```python
from build123d import *

# Parameters (mm, degrees)
F1_DEPTH = 405
F2_R     = 2.5
F2_R_2   = 4
F3_DEPTH = 2.001
F4_R     = 4
F5_DEPTH = 2.001


with BuildPart() as f1:
    # F0 (on Top) → F1 (new body)
    with BuildSketch(Plane.XY):
        with BuildLine():
            Line((0, 32.7), (0, 0))
            Line((0, 0), (2, 0))
            Line((2, 0), (2, 32.2))
            Line((2, 32.2), (20, 32.2))
            Line((20, 32.2), (20, 34.2))
            Line((20, 34.2), (1.5, 34.2))
            ThreePointArc((1.5, 34.2), (0.43934, 33.76066), (0, 32.7))
        make_face()
    extrude(amount=F1_DEPTH)

    # F2 (on face) → F3 (cut, through all)
    with BuildSketch(Plane.YZ.offset(2)):
        with Locations((9, 393.5)):
            Circle(F2_R)
        with Locations((7.5, 381)):
            Circle(F2_R_2)
        with Locations((7.5, 330)):
            Circle(F2_R_2)
        with Locations((7.5, 279)):
            Circle(F2_R_2)
        with Locations((7.5, 228)):
            Circle(F2_R_2)
        with Locations((7.5, 177)):
            Circle(F2_R_2)
        with Locations((7.5, 126)):
            Circle(F2_R_2)
        with Locations((7.5, 75)):
            Circle(F2_R_2)
        with Locations((7.5, 24)):
            Circle(F2_R_2)
        with Locations((9, 11.5)):
            Circle(F2_R)
    extrude(amount=-F3_DEPTH, mode=Mode.SUBTRACT)

    # F4 (on face) → F5 (cut, through all)
    with BuildSketch(Plane.XZ.offset(-32.2)):
        with Locations((11, 393.5)):
            Circle(F4_R)
        with Locations((11, 381)):
            Circle(F4_R)
        with Locations((11, 330)):
            Circle(F4_R)
        with Locations((11, 279)):
            Circle(F4_R)
        with Locations((11, 228)):
            Circle(F4_R)
        with Locations((11, 177)):
            Circle(F4_R)
        with Locations((11, 126)):
            Circle(F4_R)
        with Locations((11, 75)):
            Circle(F4_R)
        with Locations((11, 11.5)):
            Circle(F4_R)
        with Locations((11, 24)):
            Circle(F4_R)
    extrude(amount=-F5_DEPTH, mode=Mode.SUBTRACT)


solid = f1.part
```
The listing builds one solid part. Answer for the finished solid, in the listing's coordinates (mm). A direction names the side the tool comes from. Give positions to 0.01 mm unless a question says otherwise; leave off trailing zeros. Order: outer loops, then holes, each group sorted by start corner. A loop starts at its lowest first (then second) coordinate and runs counter-clockwise, first axis right, second up.
Item 1: The part is cut by section A-A, the plane z = 228. Give the vertices of the cut face in (x, y).
From the geometry:
outline: (0, 0) - (2, 0) - (2, 3.5) - (0, 3.5) - close; (0, 11.5) - (2, 11.5) - (2, 32.2) - (7, 32.2) - (7, 34.2) - (1.5, 34.2) arc R1.5 ccw to (0, 32.7) - close; (15, 32.2) - (20, 32.2) - (20, 34.2) - (15, 34.2) - close
Item 2: Find the intervals of material crossed by probe 1 along X at (y, z) = (32.8, 330); probe 2 along X at (y, z) = (31.5, 97.5); probe 3 along Y at (x, z) = (13.5, 185), in increasing order.
From the geometry:
probe 1: x = 0 to 7, 15 to 20
probe 2: x = 0 to 2
probe 3: y = 32.2 to 34.2
Item 3: Which of the six approach directions +Z, -Z, +X, -X, +Y, -Y give full straight-line access (tool end or side, diameter ignored) to faces 4 (the face through (13.15, 33.186, 231.373)), 5 (the face through (11, 32.2, 200))?
From the geometry:
face 4: +Y, -Y
face 5: +Z, -Z, +X, -Y
Item 4: For a pull along X with two mould halves and no side action, classify faces 1 (the face through (1.014, 6.979, 180.966)), 2 (the face through (0, 17, 200)), 3 (the face through (10.133, 33.186, 71.095)) as pulls with the +X half, pulls with the -X half, needs draft (parallel to the pull), parting line crosses it, or undercut.
From the geometry:
face 1: needs draft
face 2: pulls with the -X half
face 3: undercut
Item 5: Given pin 1 Ø9 at (y, z) = (7.5, 279) entering from +X; pin 2 Ø9 at (x, z) = (11, 75) entering from -Y; pin 3 Ø5 at (y, z) = (7.5, 330) entering from -X, each flat-ended and moving along its own axis, determine where each tip first touches the part or whether it passes through.
From the geometry:
pin 1: stops at x = 2
pin 2: stops at y = 32.2
pin 3: passes through
Item 6: The part is cut by section B-B, the plane z = 100. Give the vertices of the cut face in (x, y), and give its area (3 significant figures).
From the geometry:
outline: (0, 0) - (2, 0) - (2, 32.2) - (20, 32.2) - (20, 34.2) - (1.5, 34.2) arc R1.5 ccw to (0, 32.7) - close
area: 104 mm2
